Here's how the part is built. I have some questions about the finished solid (model axes, mm). A direction names the side the tool comes from. Coordinates: 2 decimals unless noted, no trailing zeros. Order: outer loops, then holes, each group sorted by start corner. A loop starts at its lowest first (then second) coordinate and runs counter-clockwise, first axis right, second up. Notation, with made-up numbers: (87.25, -2) - (129.25, -2) arc R23 ccw to (129.25, 13) - close; hole circle Ø9 at (-5, 3.25). An arc over 180 degrees is marked (long way). Use one line per item in the form item = value. Start each with the question number.
Autodesk Inventor part; units mm, degrees
ref_plane "YZ Plane" through (0, 0, 0) normal (1, 0, 0) x (0, 1, 0)
ref_plane "XZ Plane" through (0, 0, 0) normal (0, 1, 0) x (-1, 0, 0)
ref_plane "XY Plane" through (0, 0, 0) normal (0, 0, 1) x (1, 0, 0)
sketch "Sketch1" plane through (0, 0, 0) normal (1, 0, 0) x (0, 1, 0)
  line L0 (0, 0) -> (92.075, 67.3887)
  line L1 (92.075, 67.3887) -> (92.075, 98.8649)
  line L2 (92.075, 98.8649) -> (0, 31.4761)
  line L3 (0, 31.4761) -> (0, 0)
  dimension "d0" = 53.8
  dimension "d2" = 25.4
  dimension "d3" = 92.075
extrude "Extrusion1" add sketch "Sketch1" along normal blind 25.4
sketch "Sketch3" plane through (0, 0, 0) normal (0, -1, 0) x (1, 0, 0)
  line L0 (22.225, 28.3011) -> (3.175, 28.3011)
  line L1 (3.175, 28.3011) -> (3.175, 3.175)
  line L2 (3.175, 3.175) -> (22.225, 3.175)
  line L3 (22.225, 3.175) -> (22.225, 28.3011)
  line L4 (0, 31.4761) -> (25.4, 31.4761)
  line L5 (25.4, 0) -> (25.4, 67.3887)
  line L6 (0, 0) -> (25.4, 0)
  dimension "d10" = 19.05
  dimension "d12" = 3.175
  dimension "d13" = 3.175
  dimension "d16" = 3.175
sketch3d "3D Sketch1"
  line L0 (25.4, 0, 31.4761) -> (25.4, 92.075, 98.8649)
sweep "Sweep2" cut profiles "Sketch3" path "3D Sketch1"
properties part number "Arm Platform Diagonal strut"
1) Suppose I cut it at A-A, the plane x = 17.25. List the corners of the cut face in (y, z) for me (3 decimals).
2) For pin 1 (8 mm diameter, centred on x = 5, z = 39, fed in from -Y); pin 2 (6 mm diameter, centred on x = 13, y = 13.5, fed in from +Z); pin 3 (8 mm diameter, centred on x = 11, z = 41, fed in from -Y), each with a flat end and sliding along its axis, tell me the tip position at first contact or that it passes through.
3) Suppose I cut it at D-D, the plane z = 24.5. List the corners of the cut face in (x, y) for me (3 decimals).
4) Which directions (+Z, -Z, +X, -X, +Y, -Y) give clear straight access to the entire face, cutting with the end or side of a thin tool? Please do faces 5 (the flat face through (24, 92.075, 83)), 6 (the flat face through (12.833, 46.682, 62.467)).
5) If we mould it in two halves opening along X, with no side actions, what happens to faces 1 (the flat face through (25.4, 46, 50)), 2 (the flat face through (22.225, 43, 49)), 3 (the flat face through (12.52, 46.68, 65.64)), 4 (the flat face through (3.175, 50, 50))? For each: pulls with the +X half, pulls with the -X half, needs draft (parallel to the pull), parting line crosses it, or undercut.
6) I need wall thicknesses on probe 1 along X at (y, z) = (36, 41.5) (3 decimals); probe 2 along Z at (x, y) = (20.75, 24.5); probe 3 along Y at (x, z) = (4, 31.5). Which ranges of each line are inside material? Lowest first, please. Write a range as [from, to].
7) Suppose I cut it at C-C, the plane z = 42. List the corners of the cut face in (x, y) for me (3 decimals), then the cut area to 3 significant figures.
8) Suppose I cut it at B-B, the plane y = 15. List the corners of the cut face in (x, z) for me (3 decimals).
From the geometry:
q1.outline = (0, 0) - (92.075, 67.389) - (92.075, 70.564) - (0, 3.175) - close; (0, 28.301) - (92.075, 95.69) - (92.075, 98.865) - (0, 31.476) - close
q2.pin_1 = 4.81
q2.pin_2 = 43.55
q2.pin_3 = 7.55
q3.outline = (0, 0) - (3.175, 0) - (3.175, 29.137) - (22.225, 29.137) - (22.225, 0) - (25.4, 0) - (25.4, 33.475) - (0, 33.475) - close
q4.face_5 = +Z, -Z, +X, -X, +Y
q4.face_6 = none
q5.face_1 = pulls with the +X half
q5.face_2 = undercut
q5.face_3 = needs draft
q5.face_4 = undercut
q6.probe_1 = [0, 3.175], [22.225, 25.4]
q6.probe_2 = [17.93, 21.11], [46.23, 49.41]
q6.probe_3 = [0.03, 4.37], [38.7, 43.04]
q7.outline = (0, 14.379) - (25.4, 14.379) - (25.4, 57.386) - (0, 57.386) - close; hole (3.175, 18.717) - (22.225, 18.717) - (22.225, 53.048) - (3.175, 53.048) - close
q7.area = 438 mm2
q8.outline = (0, 10.978) - (25.4, 10.978) - (25.4, 42.454) - (0, 42.454) - close; hole (3.175, 14.153) - (22.225, 14.153) - (22.225, 39.279) - (3.175, 39.279) - close
